The listing builds one solid part. Answer for the finished solid, in the listing's coordinates (mm). A direction names the side the tool comes from. Give positions to 0.01 mm unless a question says otherwise; leave off trailing zeros. Order: outer loops, then holes, each group sorted by start corner. A loop starts at its lowest first (then second) coordinate and runs counter-clockwise, first axis right, second up. Notation, with made-up numbers: (42, -29.5) - (51, -29.5) arc R27 cw to (51, -5.5) - close; hole circle Ø2 at (81, -16). An arc over 180 degrees is marked (long way). Answer as CSV lines item,"result". Start each with the question number.
1. Determine the mould class of faces 1 (the flat face through (175, 35, -140)), 2 (the flat face through (139, 6, -88)), 3 (the cylindrical face through (173.52, 52.83, -129.75)), 4 (the flat face through (139, 11, -83.75)) for opening direction Z: +Z half, -Z half, draft (parallel to the pull), parting line (faces both ways), or undercut.
2. Consider line 1 along Y through (x, z) = (121, -104); line 2 along Y through (x, z) = (113, -86.5); line 3 along Y through (x, z) = (169.5, -115). Determine where each line is inside the solid, lowest interval first. Write a range as [from, to].
3. Section B-B on y = 42 is taken. Give the vertices of the cut face in (x, z), and give its area (3 significant figures).
4. Section C-C on x = 114 is taken. Give the vertices of the cut face in (y, z).
5. Section A-A on z = -137 is taken. Give the vertices of the cut face in (x, y), and give its area (3 significant figures).
6. Section D-D on y = 25 is taken. Give the vertices of the cut face in (x, z), and give its area (3 significant figures).
7. Which of the six approach directions +Z, -Z, +X, -X, +Y, -Y give full straight-line access (tool end or side, diameter ignored) to faces 5 (the flat face through (175, 17.5, -118)), 6 (the flat face through (139.122, 3.042, -90.756)), 7 (the flat face through (175, 31, -135)), 8 (the flat face through (169.2, 33, -120)), 9 (the flat face through (139.122, 3.042, -136.744))?
8. Flat-ended cylindrical pins translate along their axes: pin 1 (12 mm diameter, centred on x = 173, y = 32, fed in from -Z); pin 2 (4.5 mm diameter, centred on x = 99, y = 25, fed in from -Z); pin 3 (3 mm diameter, centred on y = 47.5, z = -131, fed in from +X); pin 4 (8.5 mm diameter, centred on y = 25, z = -97.5, fed in from +X). Find the tip coordinate at first contact, or state that the pin passes through.
from build123d import *

# Parameters (mm, degrees)
SKETCH1_W              = 196
SKETCH1_H              = 150
BOSS_EXTRUDE1_DEPTH    = 15
SKETCH2_W              = 166
SKETCH2_H              = 55
CUT_EXTRUDE1_DEPTH     = 9.68
SKETCH3_R              = 1.5
BOSS_EXTRUDE2_DEPTH    = 10
SKETCH4_W              = 10.9
SKETCH4_H              = 64
BOSS_EXTRUDE3_DEPTH    = 40
CUT_EXTRUDE2_DEPTH     = 109
SKETCH6_R              = 1.4
SKETCH6_R_2            = 1.375
BOSS_EXTRUDE4_DEPTH    = 10
FILLET1_R              = 10
CUT_EXTRUDE4_START     = -15
CUT_EXTRUDE4_OUTLINE_R = 1.5
CUT_EXTRUDE4_DEPTH     = 15
SKETCH10_W             = 60
SKETCH10_H             = 37
CUT_EXTRUDE5_DEPTH     = 83
SKETCH11_W             = 10
SKETCH11_H             = 52.5
CUT_EXTRUDE6_DEPTH     = 36
SKETCH13_W             = 28
SKETCH13_H             = 42.5
CUT_EXTRUDE7_DEPTH     = 19
SKETCH19_W             = 4
SKETCH19_H             = 55
SKETCH19_W_2           = 2.77
SKETCH19_H_2           = 50
CUT_EXTRUDE9_DEPTH     = 76
SKETCH21_W             = 86.997648927
SKETCH21_H             = 15
BOSS_EXTRUDE6_DEPTH    = 3.75
SKETCH22_W             = 86.997648927
SKETCH22_H             = 15
BOSS_EXTRUDE7_DEPTH    = 3.75
CUT_EXTRUDE11_DEPTH    = 94.75
CUT_EXTRUDE12_DEPTH    = 16


# Read off the part's stored shape, not the designer's step: Cut-Extrude4
with BuildPart() as part:
    # Sketch1 → Boss-Extrude1 (new body)
    with BuildSketch(Plane(origin=(0, 0, 0), x_dir=(1, 0, 0), z_dir=(0, 1, 0))):
        with Locations((98, 75)):
            Rectangle(SKETCH1_W, SKETCH1_H)
    extrude(amount=BOSS_EXTRUDE1_DEPTH)

    # Sketch2 → Cut-Extrude1 (cut)
    with BuildSketch(Plane(origin=(0, 15, 0), x_dir=(1, 0, 0), z_dir=(0, 1, 0))):
        with Locations((98, 42.5)):
            Rectangle(SKETCH2_W, SKETCH2_H)
    extrude(amount=-CUT_EXTRUDE1_DEPTH, mode=Mode.SUBTRACT)

    # Sketch3 → Boss-Extrude2 (add)
    with BuildSketch(Plane(origin=(0, 15, 0), x_dir=(1, 0, 0), z_dir=(0, 1, 0))):
        with Locations(Location((25, 133.2, 0), (0, 0, 90))):
            Circle(SKETCH3_R)
        with Locations(Location((23.7, 85, 0), (0, 0, 90))):
            Circle(SKETCH3_R)
        with Locations(Location((75.8, 118, 0), (0, 0, 90))):
            Circle(SKETCH3_R)
        with Locations(Location((75.8, 90.1, 0), (0, 0, 90))):
            Circle(SKETCH3_R)
    extrude(amount=BOSS_EXTRUDE2_DEPTH)

    # Sketch4 → Boss-Extrude3 (add)
    with BuildSketch(Plane(origin=(0, 15, 0), x_dir=(1, 0, 0), z_dir=(0, 1, 0))):
        with Locations((99.65, 108)):
            Rectangle(SKETCH4_W, SKETCH4_H)
        with Locations((174.65, 108)):
            Rectangle(SKETCH4_W, SKETCH4_H)
    extrude(amount=BOSS_EXTRUDE3_DEPTH)

    # Sketch5 → Cut-Extrude2 (cut)
    with BuildSketch(Plane(origin=(196, 0, 0), x_dir=(0, 0, -1), z_dir=(1, 0, 0))):
        Polygon((140, 55), (92.329856296, 15), (75, 15), (75, 55), align=None)
    extrude(amount=-CUT_EXTRUDE2_DEPTH, mode=Mode.SUBTRACT)

    # Sketch6 → Boss-Extrude4 (add)
    with BuildSketch(Plane(origin=(0, -36.661217825, -30.762414355), x_dir=(1, 0, 0), z_dir=(0, 0.7660444431189771, 0.6427876096865404))):
        with Locations(Location((174.7, 132.599540569, 0), (0, 0, 90))):
            Circle(SKETCH6_R)
        with Locations(Location((174.7, 101.689540569, 0), (0, 0, 90))):
            Circle(SKETCH6_R)
        with Locations(Location((99.7, 132.599540569, 0), (0, 0, 90))):
            Circle(SKETCH6_R_2)
        with Locations(Location((99.7, 101.689540569, 0), (0, 0, 90))):
            Circle(SKETCH6_R_2)
    extrude(amount=BOSS_EXTRUDE4_DEPTH)

    # Fillet1
    fillet1_edges = [part.edges().sort_by_distance(p)[0] for p in [
        (196, 15, -75),
        (98, 15, -150),
        (0, 15, -75),
        (98, 15, 0),
    ]]
    fillet(fillet1_edges, radius=FILLET1_R - 0.0001)  # a hair under: the kernel refuses the full size

    # Cut-Extrude4 outline → Cut-Extrude4 (cut)
    with BuildSketch(Plane(origin=(0, 15, 0), x_dir=(1, 0, 0), z_dir=(0, 1, 0)).offset(CUT_EXTRUDE4_START)):
        Polygon((92.232351073, 87.5), (92.232351073, 140), (196, 140), (196, 150), (0, 150), (0, 0), (196, 0), (196, 87.5), align=None)
        with Locations((23.7, 85)):
            Circle(CUT_EXTRUDE4_OUTLINE_R, mode=Mode.SUBTRACT)
        with Locations((75.8, 90.1)):
            Circle(CUT_EXTRUDE4_OUTLINE_R, mode=Mode.SUBTRACT)
        with Locations((25, 133.2)):
            Circle(CUT_EXTRUDE4_OUTLINE_R, mode=Mode.SUBTRACT)
        with Locations((75.8, 118)):
            Circle(CUT_EXTRUDE4_OUTLINE_R, mode=Mode.SUBTRACT)
    extrude(amount=CUT_EXTRUDE4_DEPTH, mode=Mode.SUBTRACT)

    # Sketch10 → Cut-Extrude5 (cut)
    with BuildSketch(Plane.ZY.offset(-92.232351073)):
        with Locations((-110, 18.5)):
            Rectangle(SKETCH10_W, SKETCH10_H)
    extrude(amount=CUT_EXTRUDE5_DEPTH, mode=Mode.SUBTRACT)

    # Sketch11 → Cut-Extrude6 (cut)
    with BuildSketch(Plane(origin=(0, 15, 0), x_dir=(1, 0, 0), z_dir=(0, 1, 0))):
        with Locations((191, 113.75)):
            Rectangle(SKETCH11_W, SKETCH11_H)
    extrude(amount=-CUT_EXTRUDE6_DEPTH, mode=Mode.SUBTRACT)

    # Sketch13 → Cut-Extrude7 (cut)
    with BuildSketch(Plane.ZY.offset(-92.232351073)):
        with Locations((-126, 36.25)):
            Rectangle(SKETCH13_W, SKETCH13_H)
    extrude(amount=-CUT_EXTRUDE7_DEPTH, mode=Mode.SUBTRACT)

    # Sketch19 → Cut-Extrude9 (cut)
    with BuildSketch(Plane.XY.offset(-87.5)):
        with Locations((94.232351073, 27.5)):
            Rectangle(SKETCH19_W, SKETCH19_H)
        with Locations((184.615, 25)):
            Rectangle(SKETCH19_W_2, SKETCH19_H_2)
    extrude(amount=-CUT_EXTRUDE9_DEPTH, mode=Mode.SUBTRACT)

    # Sketch21 → Boss-Extrude6 (add)
    with BuildSketch(Plane(origin=(0, 0, -140), x_dir=(-1, 0, 0), z_dir=(0, 0, -1))):
        with Locations((-139.731175537, 7.5)):
            Rectangle(SKETCH21_W, SKETCH21_H)
    extrude(amount=BOSS_EXTRUDE6_DEPTH)

    # Sketch22 → Boss-Extrude7 (add)
    with BuildSketch(Plane.XY.offset(-87.5)):
        with Locations((139.731175537, 7.5)):
            Rectangle(SKETCH22_W, SKETCH22_H)
    extrude(amount=BOSS_EXTRUDE7_DEPTH)

    # Sketch23 → Cut-Extrude11 (cut)
    with BuildSketch(Plane.ZY.offset(-96.232351073)):
        Polygon((-143.75, 6), (-135.035898385, 6), (-138.5, 0), (-143.75, 0), align=None)
        Polygon((-83.75, 0), (-83.75, 6), (-92.464101615, 6), (-89, 0), align=None)
    extrude(amount=-CUT_EXTRUDE11_DEPTH, mode=Mode.SUBTRACT)

    # Sketch24 → Cut-Extrude12 (cut)
    with BuildSketch(Plane(origin=(180.1, 0, 0), x_dir=(0, 0, -1), z_dir=(1, 0, 0))):
        Polygon((135, 45), (102.226776204, 17.5), (135, 17.5), align=None)
    extrude(amount=-CUT_EXTRUDE12_DEPTH, mode=Mode.SUBTRACT)


solid = part.part
Checks:
1,face 1,"-Z half"
1,face 2,"draft"
1,face 3,"undercut"
1,face 4,"+Z half"
2,line 1,"y = [0, 15]"
2,line 2,"y = [6, 15]"
2,line 3,"y = [0, 17.5], [28.22, 34.02]"
3,outline,"(169.2, -140) - (180.1, -140) - (180.1, -135) - (169.2, -135) - close; (169.2, -131.42) - (180.1, -131.42) - (180.1, -124.51) - (169.2, -124.51) - close"
3,area,"130 mm²"
4,outline,"(0, -138.5) - (6, -135.04) - (6, -143.75) - (15, -143.75) - (15, -83.75) - (6, -83.75) - (6, -92.46) - (0, -89) - close"
5,outline,"(96.23, 0) - (183.23, 0) - (183.23, 2.6) - (96.23, 2.6) - close; (96.23, 6) - (183.23, 6) - (183.23, 15) - (180.1, 15) - (180.1, 52.48) - (169.2, 52.48) - (169.2, 15) - (96.23, 15) - close"
5,area,"1,420 mm²"
6,outline,"(96.23, -112) - (105.1, -112) - (105.1, -104.25) - (96.23, -104.25) - close; (169.2, -140) - (180.1, -140) - (180.1, -135) - (169.2, -135) - close; (169.2, -111.16) - (180.1, -111.16) - (180.1, -104.25) - (169.2, -104.25) - close"
6,area,"199 mm²"
7,face 5,"+X"
7,face 6,"+Z, +X, -X"
7,face 7,"+X, -X"
7,face 8,"+Z, -Z, +Y"
7,face 9,"-Z, +X, -X"
8,pin 1,"stops at z = -140"
8,pin 2,"stops at z = -112"
8,pin 3,"stops at x = 180.1"
8,pin 4,"passes through"
